```python
from build123d import *

# Parameters (mm, degrees)
PAD_DEPTH = 2


with BuildPart() as part:
    # Sketch → Pad (new body)
    with BuildSketch(Plane.XY):
        with BuildLine():
            ThreePointArc((-25.14228, 14.122309), (-34.314711, 12.50691), (-38.960225, 4.4346))
            ThreePointArc((-38.960225, 4.4346), (-38.334534, 2.331994), (-36.445064, 1.21739))
            ThreePointArc((-19.218733, -12.375098), (-26.062582, -3.336524), (-36.445064, 1.21739))
            ThreePointArc((-19.218733, -12.375098), (-18.418224, -13.487369), (-17.206581, -14.127592))
            ThreePointArc((-12.723117, -16.130275), (-14.882343, -14.944224), (-17.206581, -14.127592))
            ThreePointArc((-12.723117, -16.130275), (-10.318463, -16.533254), (-8.408728, -15.017448))
            ThreePointArc((4.346508, -7.504289), (-3.105363, -9.437089), (-8.408728, -15.017448))
            ThreePointArc((4.346508, -7.504289), (5.513399, -7.299154), (6.509873, -6.658253))
            ThreePointArc((23.982965, -3.122935), (14.727871, -2.327704), (6.509873, -6.658253))
            ThreePointArc((23.982965, -3.122935), (25.451337, -3.302873), (26.827171, -2.759206))
            ThreePointArc((33.472919, 0.532469), (30.01349, -0.837668), (26.827171, -2.759206))
            ThreePointArc((33.472919, 0.532469), (35.549324, 2.84038), (34.47019, 5.751287))
            ThreePointArc((34.47019, 5.751287), (30.959282, 7.688022), (27.006326, 8.359998))
            ThreePointArc((27.006326, 8.359998), (13.164565, 22.80365), (-6.112904, 17.456446))
            ThreePointArc((-6.112904, 17.456446), (-16.329844, 19.797437), (-25.14228, 14.122309))
        make_face()
    extrude(amount=PAD_DEPTH)


solid = part.part
```
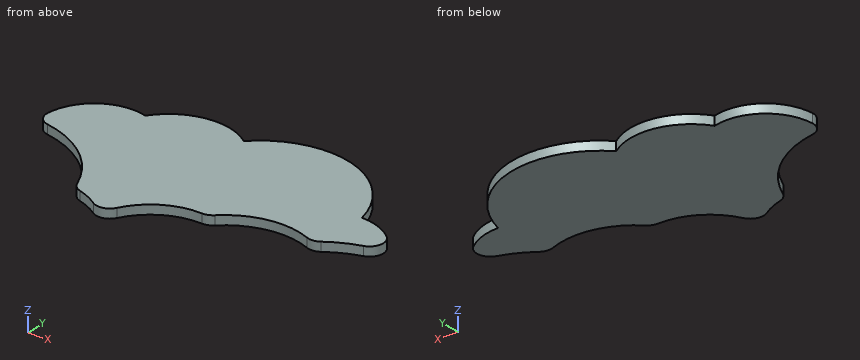
Design review of the part built by this model. Coordinates are the model's own, in mm. Round coordinates to 2 decimals unless told otherwise and drop trailing zeros. Order: outer loops, then holes, each group sorted by start corner. A loop starts at its lowest first (then second) coordinate and runs counter-clockwise, first axis right, second up. Notation, with made-up numbers: (66, -1.75) - (119, -1.75) arc R30 cw to (119, 22.25) - close; hole circle Ø10 at (89, -28.75). An arc over 180 degrees is marked (long way). Return JSON: item names as keys, results as strings.
Q1. Consider section D-D on x = -2.5. Write out the cut boundary in (y, z).
Computed values:
{"outline": "(-9.1, 0) - (20.43, 0) - (20.43, 2) - (-9.1, 2) - close"}
Q2. Consider section A-A on y = 18.5. Write out the cut boundary in (x, z).
Computed values:
{"outline": "(-20.18, 0) - (-7.82, 0) - (-7.82, 2) - (-20.18, 2) - close; (-5.04, 0) - (21.04, 0) - (21.04, 2) - (-5.04, 2) - close"}
Q3. Consider section B-B on z = 1.5. Write out the cut boundary in (x, y), plus the area to 3 significant figures.
Computed values:
{"outline": "(-38.96, 4.43) arc R3 ccw to (-36.45, 1.22) arc R22.5 cw to (-19.22, -12.38) arc R3 ccw to (-17.21, -14.13) arc R15 cw to (-12.72, -16.13) arc R3 ccw to (-8.41, -15.02) arc R14 cw to (4.35, -7.5) arc R3 ccw to (6.51, -6.66) arc R16.5 cw to (23.98, -3.12) arc R3 ccw to (26.83, -2.76) arc R22.5 cw to (33.47, 0.53) arc R3 ccw to (34.47, 5.75) arc R12 ccw to (27.01, 8.36) arc R19.5 ccw to (-6.11, 17.46) arc R13.5 ccw to (-25.14, 14.12) arc R11 ccw to start", "area": "1,690 mm2"}
Q4. For pin 1 Ø2 at (x, y) = (-25, 16) entering from -Z; pin 2 Ø1 at (x, z) = (18.5, 0.5) entering from +Y, all flat-tipped, find the tip position at first contact; note any pin that passes through.
Computed values:
{"pin 1": "passes through", "pin 2": "stops at y = 20.74"}
Q5. Wall thickness on L1, parallel to X at y = 5.5, z = 1.5; L2, parallel to Y at x = -4, z = 1.9; L3, parallel to Y at x = 13, z = 0.85: over which ranges is each line inside the solid? List them lowest first. Write a range as [from, to].
Computed values:
{"L1": "x = [-38.82, 34.75]", "L2": "y = [-10.01, 19.37]", "L3": "y = [-2.78, 22.85]"}
Q6. Consider section C-C on y = 7. Write out the cut boundary in (x, z), plus the area to 3 significant figures.
Computed values:
{"outline": "(-38.43, 0) - (32.55, 0) - (32.55, 2) - (-38.43, 2) - close", "area": "142 mm2"}
